Model file for the job. Use its own axes, mm. A direction names the side the tool comes from. Coordinates: 2 decimals unless noted, no trailing zeros. Loops run counter-clockwise (first coordinate to the right, second up) from the corner with the lowest first, then second, coordinate; pieces in that order, holes last.
from build123d import *

# Parameters (mm, degrees)
SKETCH_1_R          = 4
EXTRUDE_1_DEPTH     = 7
SKETCH_2_R          = 1.6
CUT_EXTRUDE_1_DEPTH = 10
SKETCH_3_OUTSIDE_W  = 12.66
SKETCH_3_OUTSIDE_H  = 12.66
SKETCH_3_OUTSIDE_R  = 3
CUT_EXTRUDE_2_DEPTH = 4
SKETCH_4_R          = 4
SKETCH_4_R_2        = 1.6
EXTRUDE_2_DEPTH     = 3
SKETCH_5_R          = 4
SKETCH_5_R_2        = 3
CUT_EXTRUDE_3_DEPTH = 2.1
SKETCH_6_OUTSIDE_W  = 13.02
SKETCH_6_OUTSIDE_H  = 13.02
SKETCH_6_OUTSIDE_R  = 3
CUT_EXTRUDE_4_DEPTH = 7
SKETCH_7_R          = 3
CUT_EXTRUDE_5_DEPTH = 2.8


with BuildPart() as part:
    # 草图1 → 凸台-拉伸1 (new body)
    with BuildSketch(Plane.XY):
        Circle(SKETCH_1_R)
    extrude(amount=EXTRUDE_1_DEPTH)

    # 草图2 → 切除-拉伸1 (cut, through all)
    with BuildSketch(Plane.XY.offset(7)):
        Circle(SKETCH_2_R)
    extrude(amount=-CUT_EXTRUDE_1_DEPTH, mode=Mode.SUBTRACT)

    # 草图3 outside → 切除-拉伸2 (cut)
    with BuildSketch(Plane.XY.offset(7)):
        Rectangle(SKETCH_3_OUTSIDE_W, SKETCH_3_OUTSIDE_H)
        Circle(SKETCH_3_OUTSIDE_R, mode=Mode.SUBTRACT)
    extrude(amount=-CUT_EXTRUDE_2_DEPTH, mode=Mode.SUBTRACT)

    # 草图4 → 凸台-拉伸2 (add)
    with BuildSketch(Plane.XY.offset(7)):
        Circle(SKETCH_4_R)
        Circle(SKETCH_4_R_2, mode=Mode.SUBTRACT)
    extrude(amount=EXTRUDE_2_DEPTH)

    # 草图5 → 切除-拉伸3 (cut, symmetric)
    with BuildSketch(Plane.XY.offset(5)):
        Circle(SKETCH_5_R)
        Circle(SKETCH_5_R_2, mode=Mode.SUBTRACT)
    extrude(amount=CUT_EXTRUDE_3_DEPTH, both=True, mode=Mode.SUBTRACT)

    # 草图6 outside → 切除-拉伸4 (cut)
    with BuildSketch(Plane(origin=(0, 0, 0), x_dir=(-1, 0, 0), z_dir=(0, 0, -1))):
        Rectangle(SKETCH_6_OUTSIDE_W, SKETCH_6_OUTSIDE_H)
        with Locations(Location((0, 0, 0), (0, 0, 180))):
            Circle(SKETCH_6_OUTSIDE_R, mode=Mode.SUBTRACT)
    extrude(amount=-CUT_EXTRUDE_4_DEPTH, mode=Mode.SUBTRACT)

    # 草图7 → 切除-拉伸5 (cut)
    with BuildSketch(Plane(origin=(0, 0, 0), x_dir=(-1, 0, 0), z_dir=(0, 0, -1))):
        with Locations(Location((0, 0, 0), (0, 0, 180))):
            Circle(SKETCH_7_R)
    extrude(amount=-CUT_EXTRUDE_5_DEPTH, mode=Mode.SUBTRACT)


solid = part.part
Q1. Slice it at D-D (y = -2.25). List the corners of the cut face in (x, z).
Answers:
outline: (-3.31, 7.1) - (-1.98, 7.1) - (-1.98, 2.8) - (1.98, 2.8) - (1.98, 7.1) - (3.31, 7.1) - (3.31, 10) - (-3.31, 10) - close
Q2. Slice it at A-A (y = 0). List the corners of the cut face in (x, z).
Answers:
outline: (-4, 7.1) - (-3, 7.1) - (-3, 2.8) - (-1.6, 2.8) - (-1.6, 10) - (-4, 10) - close; (1.6, 2.8) - (3, 2.8) - (3, 7.1) - (4, 7.1) - (4, 10) - (1.6, 10) - close
Q3. Drill centre lines: line 1 (Y direction, x = 0, z = 9.35); line 2 (Y direction, x = 0, z = 5.3); line 3 (X direction, y = 1.25, z = 3.5). Where is each one in solid material? Low to high.
Answers:
line 1: y = -4 to -1.6, 1.6 to 4
line 2: y = -3 to -1.6, 1.6 to 3
line 3: x = -2.73 to -1, 1 to 2.73
Q4. Which spindle directions (+Z, -Z, +X, -X, +Y, -Y) get a long thin tool onto all of the face, cutting with end or side? Do faces 1 (the flat face through (2, 0, 10)), 2 (the flat face through (1, 3, 7.1)). Say none if no direction does.
Answers:
face 1: +Z, +X, -X, +Y, -Y
face 2: -Z
Q5. Flat gauge pins, fed straight in: P1, Ø2, axis at y = -1, z = 4, coming from the -X side; P2, Ø3, axis at y = 3, z = 5, coming from the -X side. Where does each tip first touch, or does it go through?
Answers:
P1: stops at x = -3
P2: stops at x = -2.6
Q6. Slice it at C-C (z = 8.25). List the corners of the cut face in (x, y), and give its area (3 significant figures).
Answers:
outline: circle Ø8 at (0, 0); hole circle Ø3.2 at (0, 0)
area: 42.2 mm2
